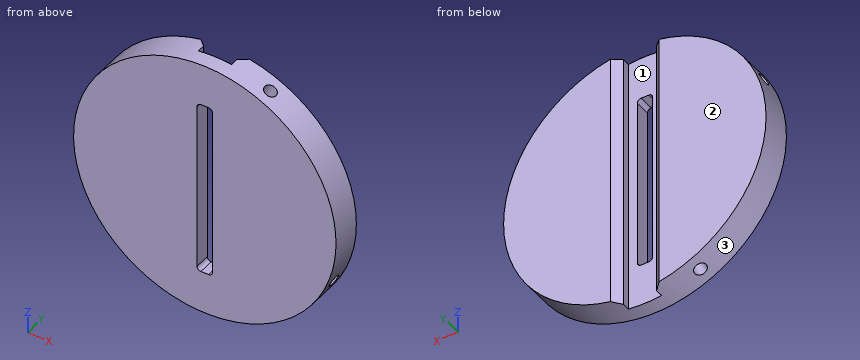
```python
from build123d import *

# Parameters (mm, degrees)
SKETCH1_R           = 17
BOSS_EXTRUDE1_DEPTH = 4
SKETCH23_W          = 4.3
SKETCH23_H          = 36
CUT_EXTRUDE5_DEPTH  = 2
SKETCH24_W          = 2
SKETCH24_H          = 23
CUT_EXTRUDE6_DEPTH  = 25.124676164
FILLET4_R           = 0.5
CHAMFER1_SIZE       = 1
CIRPATTERN1_COUNT   = 4


with BuildPart() as part:
    # Sketch1 → Boss-Extrude1 (new body)
    with BuildSketch(Plane(origin=(0, 0, 0), x_dir=(1, 0, 0), z_dir=(0, 1, 0))):
        with Locations(Location((0, 0, 0), (0, 0, 270))):
            Circle(SKETCH1_R)
    extrude(amount=BOSS_EXTRUDE1_DEPTH)

    # Sketch23 → Cut-Extrude5 (cut)
    with BuildSketch(Plane(origin=(0, 4, 0), x_dir=(1, 0, 0), z_dir=(0, 1, 0))):
        with Locations((0, -0.174485126)):
            Rectangle(SKETCH23_W, SKETCH23_H)
    extrude(amount=-CUT_EXTRUDE5_DEPTH, mode=Mode.SUBTRACT)

    # Sketch24 → Cut-Extrude6 (cut, through all)
    with BuildSketch(Plane(origin=(0, 2, 0), x_dir=(1, 0, 0), z_dir=(0, 1, 0))):
        Rectangle(SKETCH24_W, SKETCH24_H)
    extrude(amount=-CUT_EXTRUDE6_DEPTH, mode=Mode.SUBTRACT)

    # Fillet4
    fillet4_edges = [part.edges().sort_by_distance(p)[0] for p in [
        (1, 1, -11.5),
        (1, 1, 11.5),
        (-1, 1, 11.5),
        (-1, 1, -11.5),
    ]]
    fillet(fillet4_edges, radius=FILLET4_R)

    # Chamfer1
    chamfer1_edges = [part.edges().sort_by_distance(p)[0] for p in [
        (-2.15, 4, 0),
        (2.15, 4, 0),
    ]]
    chamfer(chamfer1_edges, length=CHAMFER1_SIZE)

    # Sketch27 → M2 Tapped Hole1 (revolve, cut)
    with BuildSketch(Plane(origin=(-7.18451045, 2, -15.40723238), x_dir=(-0.9063077870366497, 0, 0.4226182617407), z_dir=(0, 1, 0))):
        Polygon((0, 0), (0, 5.680688495), (0.8, 5.2), (0.8, 0), align=None)
    m2_tapped_hole1 = revolve(axis=Axis((-9.868136412, 2, -21.162286827), (0.42261826174069994, 0, 0.9063077870366498)), mode=Mode.SUBTRACT)

    # CirPattern1: M2 Tapped Hole1 ×4 about axis
    cirpattern1_axis = Axis((0, 0, 0), (0, -1, 0))
    for i in range(1, CIRPATTERN1_COUNT):
        add(m2_tapped_hole1.rotate(cirpattern1_axis, i * 360 / CIRPATTERN1_COUNT), mode=Mode.SUBTRACT)


solid = part.part
```
Could you check a few things on this model? Use its own coordinates, in mm. Face numbers are marked on the shaded views. Give positions to 0.01 mm unless a question says otherwise; leave off trailing zeros. Loops run counter-clockwise (first coordinate to the right, second up) from the corner with the lowest first, then second, coordinate; pieces in that order, holes last. Notation, with made-up numbers: (-16.75, 0.25) - (29.25, 0.25) arc R25 cw to (29.25, 39.25) - close; hole circle Ø10 at (69.5, -8). An arc over 180 degrees is marked (long way). Answer in a Markdown table with one row per item. Add a question column.
Q1. If we section it at C-C (y = 3.5): List the corners of the cut face in (x, z) for me.
Q2. Please list where these lines run through material, in increasing order: L1, parallel to X at y = 1.55, z = -6.5; L2, parallel to X at y = 2.5, z = 5; L3, parallel to Z at x = -0.5, y = 0.95. Write a range as from..to.
Q3. We'd pull the mould along X, two halves only. Please class the marked faces 1, 2 and 3: +X half, -X half, draft (parallel to the pull), parting line (faces both ways), or undercut.
Q4. For pin 1 (1 mm diameter, centred on x = -5, y = 1, fed in from +Z); pin 2 (1.6 mm diameter, centred on y = 1, z = 3, fed in from +X); pin 3 (1.6 mm diameter, centred on y = 1, z = -4.5, fed in from -X), each with a flat end and sliding along its axis, tell me the tip position at first contact or that it passes through.
Q5. If we section it at A-A (z = 0): List the corners of the cut face in (x, y) for me.
Q6. If we section it at B-B (x = 0): List the corners of the cut face in (y, z) for me.
The answers:
| question | item | result |
|---|---|---|
| 1 | outline | (-2.65, -16.79) - (-2.65, 16.79) arc R17 ccw to start; (2.65, -16.79) arc R17 ccw to (2.65, 16.79) - close |
| 2 | L1 | x = -15.71..-1, 1..12.37, 15.5..15.71 |
| 2 | L2 | x = -16.25..-12.2, -10.5..-2.15, 2.15..16.25 |
| 2 | L3 | z = -16.99..-11.5, 11.5..16.99 |
| 3 | face 1 | undercut |
| 3 | face 2 | draft |
| 3 | face 3 | parting line |
| 4 | pin 1 | stops at z = 16.39 |
| 4 | pin 2 | stops at x = 16.86 |
| 4 | pin 3 | stops at x = -16.59 |
| 5 | outline | (-17, 0) - (-1, 0) - (-1, 2) - (-2.15, 2) - (-2.15, 3) - (-3.15, 4) - (-17, 4) - close; (1, 0) - (17, 0) - (17, 4) - (3.15, 4) - (2.15, 3) - (2.15, 2) - (1, 2) - close |
| 6 | outline | (0, -17) - (2, -17) - (2, -11.5) - (0, -11.5) - close; (0, 11.5) - (2, 11.5) - (2, 17) - (0, 17) - close |
